Design review of the part shown in the three views and the two pictorial views. Dimensions are in mm from the part's minimum x, y and z. A direction names the side the tool comes from. Round coordinates to 2 decimals unless told otherwise and drop trailing zeros. Order: outer loops, then holes, each group sorted by start corner. A loop starts at its lowest first (then second) coordinate and runs counter-clockwise, first axis right, second up. Notation, with made-up numbers: M 0.5,-8 L 15.5,-8 A7 cw 15.5,4 Z; hole C -20,-28.5 d4. An arc over 180 degrees is marked long. Use a Markdown table: item, result. Add a question column.
(1) Take a section at B-B (z = 11.5). Write out the cut boundary in (x, y), then the cut area to 3 significant figures.
(2) Take a section at A-A (x = 24.5). Write out the cut boundary in (y, z), then the cut area to 3 significant figures.
(3) Machinability: for the marked faces 1, 2, 3 and 4, which of the approach directions +Z, -Z, +X, -X, +Y, -Y give a long, thin tool a straight path to every point of the face, cutting with its end or side? Answer none if there is none.
(4) For pin 1 (4 mm diameter, centred on y = 17, z = 11.5, fed in from +X); pin 2 (8 mm diameter, centred on y = 28, z = 32.5, fed in from +X); pin 3 (8 mm diameter, centred on y = 44.5, z = 24.5, fed in from +X), all flat-tipped, find the tip position at first contact; note any pin that passes through.
(5) The part is to be moulded in two halves that separate along Z. For the marked faces 5, 6 and 7, say which applies: released by +Z, released by -Z, zero draft, split by the parting line, or undercut.
(6) Take a section at C-C (x = 15). Write out the cut boundary in (y, z), then the cut area to 3 significant figures.
(7) Take a section at D-D (y = 47.5). Write out the cut boundary in (x, z).
(8) To check wall thickness, follow probe 1 along Y at (x, z) = (23.5, 36); probe 2 along Z at (x, y) = (30, 6.75); probe 3 along X at (y, z) = (27.5, 23). State the ranges of each line that lie inside material, in increasing order. Write a range as from..to.
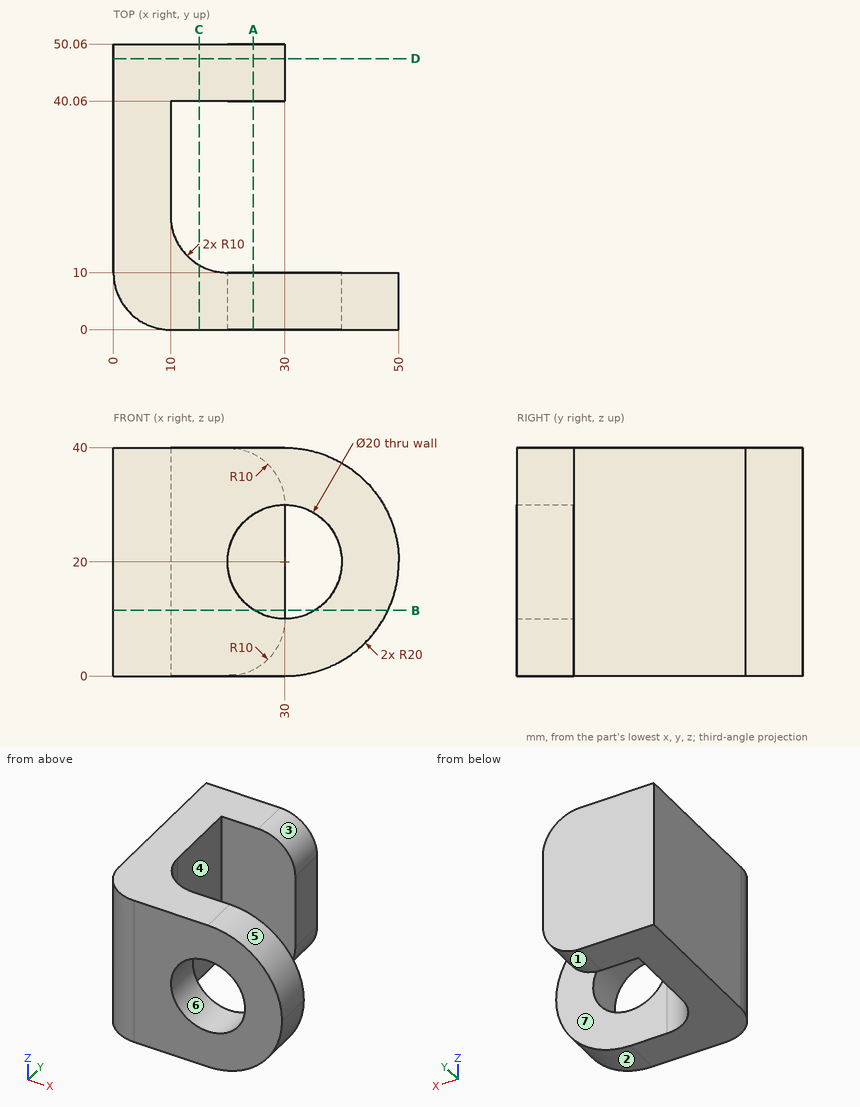
Verdict:
| question | item | result |
|---|---|---|
| 1 | outline | M 0,10 A10 ccw 10,0 L 24.73,0 L 24.73,10 L 20,10 A10 cw 10,20 L 10,40.06 L 30,40.06 L 30,50.06 L 0,50.06 Z; M 35.27,0 L 48.1,0 L 48.1,10 L 35.27,10 Z |
| 1 | area | 976 mm^2 |
| 2 | outline | M 0,0 L 10,0 L 10,11.65 L 0,11.65 Z; M 0,28.35 L 10,28.35 L 10,40 L 0,40 Z; M 40.06,1.07 L 50.06,1.07 L 50.06,38.93 L 40.06,38.93 Z |
| 2 | area | 612 mm^2 |
| 3 | face 1 | -Z, +X, +Y |
| 3 | face 2 | -Z, +X, +Y, -Y |
| 3 | face 3 | +Z, +X, +Y |
| 3 | face 4 | +Z, -Z, +X |
| 4 | pin 1 | stops at x = 11.34 |
| 4 | pin 2 | stops at x = 10 |
| 4 | pin 3 | stops at x = 30 |
| 5 | face 5 | released by +Z |
| 5 | face 6 | undercut |
| 5 | face 7 | zero draft |
| 6 | outline | M 0,0 L 11.34,0 L 11.34,40 L 0,40 Z; M 40.06,0 L 50.06,0 L 50.06,40 L 40.06,40 Z |
| 6 | area | 854 mm^2 |
| 7 | outline | M 0,0 L 20,0 A10 ccw 30,10 L 30,30 A10 ccw 20,40 L 0,40 Z |
| 8 | probe 1 | y = 0..10, 40.06..50.06 |
| 8 | probe 2 | z = 0..10, 30..40 |
| 8 | probe 3 | x = 0..10 |
